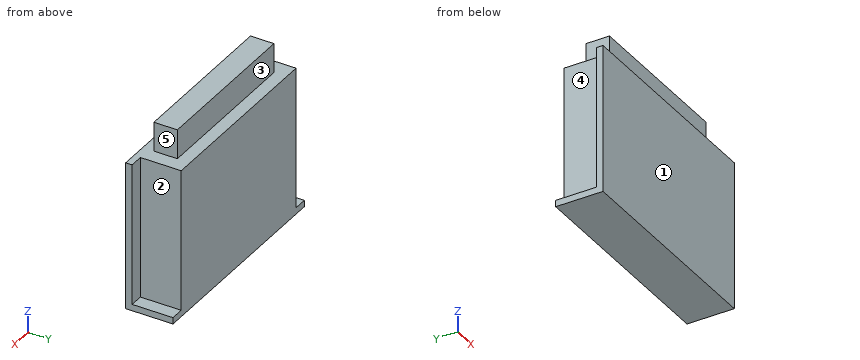
from build123d import *

# Parameters (mm, degrees)
SKETCH1_W           = 111.5
SKETCH1_H           = 75.8
BOSS_EXTRUDE1_DEPTH = 3.3
BOSS_EXTRUDE2_DEPTH = 20.9
SKETCH3_W           = 82
SKETCH3_H           = 12
BOSS_EXTRUDE3_DEPTH = 15


with BuildPart() as part:
    # Sketch1 → Boss-Extrude1 (new body)
    with BuildSketch(Plane(origin=(0, 0, 0), x_dir=(1, 0, 0), z_dir=(0, 1, 0))):
        Rectangle(SKETCH1_W, SKETCH1_H)
    extrude(amount=BOSS_EXTRUDE1_DEPTH)

    # Sketch2 → Boss-Extrude2 (add)
    with BuildSketch(Plane(origin=(0, 3.3, 0), x_dir=(1, 0, 0), z_dir=(0, 1, 0))):
        Polygon((48.75, 37.9), (-48.75, 37.9), (-55.75, 37.9), (-55.75, 34.6), (-48.75, 34.6), (-48.75, -37.9), (48.75, -37.9), (48.75, 34.6), (55.75, 34.6), (55.75, 37.9), align=None)
    extrude(amount=BOSS_EXTRUDE2_DEPTH)

    # Sketch3 → Boss-Extrude3 (add)
    with BuildSketch(Plane.XY.offset(37.9)):
        with Locations((0.25, 11.7)):
            Rectangle(SKETCH3_W, SKETCH3_H)
    extrude(amount=BOSS_EXTRUDE3_DEPTH)


solid = part.part
Input: part model. Units: mm. Frame: model coordinates. Face numbers are marked on the shaded views. A direction names the side the tool comes from. Coordinates: 2 decimals unless noted, no trailing zeros. Loops run counter-clockwise (first coordinate to the right, second up) from the corner with the lowest first, then second, coordinate; pieces in that order, holes last.
(1) Section D-D on x = 47.5. Return the cut outline in (y, z).
(2) Section A-A on y = 19.5. Return the cut outline in (x, z).
(3) Material intervals for probe 1 along X at (y, z) = (20, -23); probe 2 along X at (y, z) = (17.25, 48.5); probe 3 along Z at (x, y) = (42, 20.25), sorted ascending.
(4) Section B-B on x = 16. Return the cut outline in (y, z).
(5) Set-up query: the marked faces 1, 2, 3, 4 and 5. Return all of +Z, -Z, +X, -X, +Y, -Y with unobstructed straight access to the full face (end or side cutting, diameter ignored); none if empty.
(6) Section C-C on y = 8.25. Return the cut outline in (x, z).
(7) First-contact query: pin 1 Ø2 at (x, y) = (51.5, 17) entering from +Z; pin 2 Ø3 at (y, z) = (5, -21.5) entering from +X; pin 3 Ø5 at (y, z) = (5, -10) entering from +X; pin 4 Ø3.5 at (x, z) = (53.5, -9) entering from +Y. Flat tips, straight axial feed; report the tip coordinate or a pass-through.
Data:
1. outline: (0, -37.9) - (24.2, -37.9) - (24.2, 37.9) - (0, 37.9) - close
2. outline: (-55.75, -37.9) - (55.75, -37.9) - (55.75, -34.6) - (48.75, -34.6) - (48.75, 37.9) - (-48.75, 37.9) - (-48.75, -34.6) - (-55.75, -34.6) - close
3. probe 1: x = -48.75 to 48.75
3. probe 2: x = -40.75 to 41.25
3. probe 3: z = -37.9 to 37.9
4. outline: (0, -37.9) - (24.2, -37.9) - (24.2, 37.9) - (17.7, 37.9) - (17.7, 52.9) - (5.7, 52.9) - (5.7, 37.9) - (0, 37.9) - close
5. face 1: +Z, -Z, +X, -X, -Y
5. face 2: +Z, +X, +Y
5. face 3: +Z, +X, -X, +Y
5. face 4: +Z, -X, +Y
5. face 5: +Z, +X, +Y, -Y
6. outline: (-55.75, -37.9) - (55.75, -37.9) - (55.75, -34.6) - (48.75, -34.6) - (48.75, 37.9) - (41.25, 37.9) - (41.25, 52.9) - (-40.75, 52.9) - (-40.75, 37.9) - (-48.75, 37.9) - (-48.75, -34.6) - (-55.75, -34.6) - close
7. pin 1: stops at z = -34.6
7. pin 2: stops at x = 48.75
7. pin 3: stops at x = 55.75
7. pin 4: stops at y = 3.3
